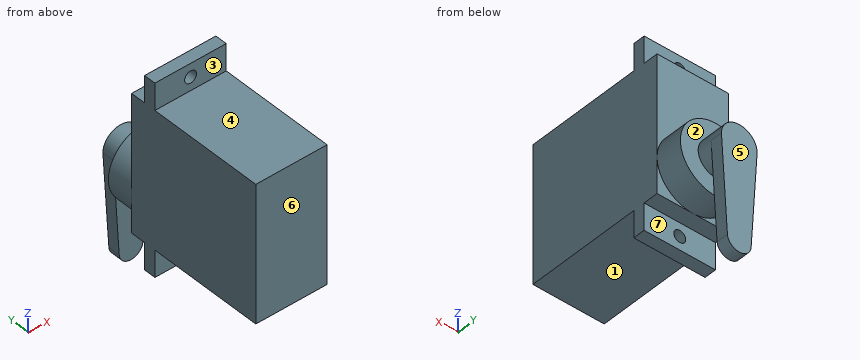
Autodesk Fusion 360 part; units mm, degrees
sketch "Boceto1" plane through (0, 0, 0) normal (0, 1, 0) x (1, 0, 0)
  line L0 (-25, 25) -> (-25, 2)
  line L1 (-25, 25) -> (-13, 25)
  line L2 (-13, 25) -> (-13, 2)
  line L3 (-25, 2) -> (-13, 2)
  dimension "d1" = 23
  dimension "d2" = 12
extrude "Extruir1" add sketch "Boceto1" along normal blind 24
sketch "Boceto2" plane through (0, 0, -2) normal (0, 0, 1) x (1, 0, 0)
  line L0 (-25, 0) -> (-13, 0)
  line L1 (-13, 0) -> (-13, 24)
  line L2 (-13, 24) -> (-25, 24)
  line L3 (-25, 24) -> (-25, 0)
  line L4 (-13, 19.5) -> (-25, 19.5)
  line L5 (-25, 19.5) -> (-25, 21.5)
  line L6 (-25, 21.5) -> (-13, 21.5)
  line L7 (-13, 21.5) -> (-13, 19.5)
  dimension "d5" = 19.5
  dimension "d6" = 2
extrude "Extruir2" add sketch "Boceto2" along normal blind 4.5 contours L1 L3 L4 L5 L6 L7
sketch "Boceto3" plane through (0, 0, -25) normal (0, 0, -1) x (-1, 0, 0)
  line L0 (13, 0) -> (25, 0)
  line L1 (25, 0) -> (25, 24)
  line L2 (25, 24) -> (13, 24)
  line L3 (13, 24) -> (13, 0)
  line L4 (25, 19.5) -> (13, 19.5)
  line L5 (13, 19.5) -> (13, 21.5)
  line L6 (13, 21.5) -> (25, 21.5)
  line L7 (25, 21.5) -> (25, 19.5)
  dimension "d9" = 19.5
  dimension "d10" = 2
extrude "Extruir3" add sketch "Boceto3" along normal blind 4.5 contours L1 L3 L4 L5 L6 L7
sketch "Boceto4" plane through (0, 21.5, 0) normal (0, 1, 0) x (-1, 0, 0)
  line L0 (13, -2) -> (25, -2)
  line L1 (25, -2) -> (25, 2.5)
  line L2 (25, 2.5) -> (13, 2.5)
  line L3 (13, 2.5) -> (13, -2)
  circle A0 centre (19, 0.25) radius 1
  dimension "d13" = 2
sketch "Boceto5" plane through (0, 21.5, 0) normal (0, 1, 0) x (-1, 0, 0)
  line L0 (25, -25) -> (13, -25)
  line L1 (13, -25) -> (13, -29.5)
  line L2 (13, -29.5) -> (25, -29.5)
  line L3 (25, -29.5) -> (25, -25)
  circle A0 centre (19, -27.25) radius 1
  dimension "d14" = 2
extrude "Extruir4" cut sketch "Boceto4" sketch "Boceto5" against normal blind 5 contours A0 of sketch 2 contours A0
sketch "Boceto6" plane through (0, 24, 0) normal (0, 1, 0) x (-1, 0, 0)
  line L0 (25, -25) -> (25, -2)
  line L1 (25, -2) -> (13, -2)
  line L2 (13, -2) -> (13, -25)
  line L3 (13, -25) -> (25, -25)
  line L4 (13, -25) -> (13, -19)
  circle A0 centre (19, -19) radius 6
extrude "Extruir5" add sketch "Boceto6" along normal blind 4.5 contours A0
sketch "Boceto7" plane through (0, 28.5, 0) normal (0, 1, 0) x (-1, 0, 0)
  circle A0 centre (19, -19) radius 6
  circle A1 centre (19, -19) radius 3
  dimension "d19" = 6
extrude "Extruir6" add sketch "Boceto7" along normal blind 2.5 contours A1
sketch "Boceto8" plane through (0, 31, 0) normal (0, 1, 0) x (-1, 0, 0)
  line L0 (22, -19) -> (20.995, -35.1418)
  line L1 (16, -19) -> (17.005, -35.1418)
  arc A0 (22, -19) -> (16, -19) centre (19, -19) ccw
  arc A1 (17.005, -35.1418) -> (20.995, -35.1418) centre (19, -35) ccw
extrude "Extruir7" add sketch "Boceto8" along normal blind 2
Work out the finished part from the listing and answer in its coordinate system (mm). Face numbers are marked on the shaded views. A direction names the side the tool comes from. Give positions to 0.01 mm unless a question says otherwise; leave off trailing zeros. Loops run counter-clockwise (first coordinate to the right, second up) from the corner with the lowest first, then second, coordinate; pieces in that order, holes last. Notation, with made-up numbers: (34.25, -12) - (66.25, -12) arc R33 ccw to (66.25, 18) - close; hole circle Ø5 at (68.25, 10.5). An arc over 180 degrees is marked (long way). One line per question, with ' | ' between items.
(1) The part is cut by section B-B (z = -27.25). Write down the section's boundary in (x, y).
Recorded:
outline: (-25, 19.5) - (-20, 19.5) - (-20, 21.5) - (-25, 21.5) - close; (-21.49, 31) - (-16.51, 31) - (-16.51, 33) - (-21.49, 33) - close; (-18, 19.5) - (-13, 19.5) - (-13, 21.5) - (-18, 21.5) - close
(2) Each of these flat-tipped pins is pushed along its axis until it touches: pin 1 Ø2 at (x, z) = (-17, 0) entering from +Y; pin 2 Ø6 at (x, y) = (-17.5, 19.5) entering from -Z; pin 3 Ø0.8 at (x, y) = (-18.5, 22.5) entering from -Z. Where does it stop, or does it pass through?
Recorded:
pin 1: stops at y = 21.5 | pin 2: stops at z = -29.5 | pin 3: stops at z = -25
(3) The part is cut by section C-C (x = -20.5). Write down the section's boundary in (y, z), then the cut area to 3 significant figures.
Recorded:
outline: (0, -25) - (19.5, -25) - (19.5, -29.5) - (21.5, -29.5) - (21.5, -25) - (24, -25) - (24, -24.81) - (28.5, -24.81) - (28.5, -21.6) - (31, -21.6) - (31, -36.32) - (33, -36.32) - (33, -16.4) - (28.5, -16.4) - (28.5, -13.19) - (24, -13.19) - (24, -2) - (21.5, -2) - (21.5, 2.5) - (19.5, 2.5) - (19.5, -2) - (0, -2) - close | area: 675 mm²
(4) The part is cut by section D-D (y = 26). Write down the section's boundary in (x, z).
Recorded:
outline: circle Ø12 at (-19, -19)
(5) Straight lines are drawn through the part: probe 1 along Z at (x, y) = (-19, 20.5); probe 2 along Y at (x, z) = (-16, -13.5); probe 3 along Y at (x, z) = (-17.75, -32). For each, find the intervals that lie inside material, in ascending order.
Recorded:
probe 1: z = -29.5 to -28.25, -26.25 to -0.75, 1.25 to 2.5 | probe 2: y = 0 to 24 | probe 3: y = 31 to 33
(6) A tool of negligible diameter and unlimited length cuts with its end or side. For the marked faces 1, 2 and 3, from which of +Z, -Z, +X, -X, +Y, -Y can it reach the whole face along a straight path? Write none if from no direction.
Recorded:
face 1: -Z, +X, -X, -Y | face 2: none | face 3: +Z, +X, -X, -Y
(7) The mould has two halves that part along Y. Classify the marked faces 4, 5, 6 and 7: +Y half, -Y half, draft (parallel to the pull), parting line (faces both ways), or undercut.
Recorded:
face 4: draft | face 5: +Y half | face 6: -Y half | face 7: undercut
(8) The part is cut by section A-A (z = 0.25). Write down the section's boundary in (x, y), then the cut area to 3 significant figures.
Recorded:
outline: (-25, 19.5) - (-20, 19.5) - (-20, 21.5) - (-25, 21.5) - close; (-18, 19.5) - (-13, 19.5) - (-13, 21.5) - (-18, 21.5) - close | area: 20.0 mm²
